Source: CAD feature listing. Evaluate the final solid. Frame: model axes, mm. A direction names the side the tool comes from. Give positions to 0.01 mm unless a question says otherwise; leave off trailing zeros. Loops run counter-clockwise (first coordinate to the right, second up) from the corner with the lowest first, then second, coordinate; pieces in that order, holes last. Notation, with made-up numbers: (19, 0.5) - (42, 0.5) arc R11 cw to (42, 9.5) - close; hole circle Ø2 at (2.25, 67.5). An arc over 180 degrees is marked (long way). Write each question's results on one line, items separated by ' | '. Start each with the question number.
(1) Reachability of faces 5 (the flat face through (20.902, 0, 2)), 6 (the flat face through (-11.536, 24, 2)), 7 (the cylindrical face through (11.998, 30.107, 1.972)), 8 (the flat face through (-27.75, 17.72, 1.97)) from +Z, -Z, +X, -X, +Y, -Y: full face, straight path, thin tool, end or side. Return the list, or none.
(2) Pull-direction query (Y, two-part tool) for faces 1 (the cylindrical face through (11.935, -30.105, 1.972)), 2 (the flat face through (-1, 1, 0)), 3 (the cylindrical face through (-36.265, -33.787, 1.972)), 4 (the cylindrical face through (-15.52, -19.77, 1.97)); classes: pulls with the +Y half, pulls with the -Y half, needs draft (parallel to the pull), parting line crosses it, or undercut.
(3) Contact query for flat-ended pins moving along their axis: pin 1 (2 mm diameter, centred on x = -3.5, z = 1.5, fed in from -Y); pin 2 (0.8 mm diameter, centred on x = -11, z = 1.5, fed in from +Y); pin 3 (0.6 mm diameter, centred on x = 10.5, z = 2, fed in from -Y). Output: stop coordinate, or through.
(4) Cut plane B-B on y = 0. Return the cut outline in (x, z).
(5) Cut plane A-A on x = 15.25. Return the cut outline in (y, z), then the cut area to 3 significant figures.
(6) Cut plane C-C on x = 5. Return the cut outline in (y, z), then the cut area to 3 significant figures.
(7) Material intervals for line 1 along X through (y, z) = (-19, 2.25); line 2 along Y through (x, z) = (-15.25, 3.1); line 3 along Y through (x, z) = (-2.5, 2.4), sorted ascending. Write a range as [from, to].
from build123d import *

# Parameters (mm, degrees)
F0_R     = 1.25
F1_DEPTH = 4


with BuildPart() as f1:
    # F0 (on Top) → F1 (new body)
    with BuildSketch(Plane.XY):
        with BuildLine():
            ThreePointArc((21.584305, 11.679198), (21.963351, 12.114397), (22.366871, 12.527004))
            Line((22.366871, 12.527004), (32.982551, 22.772845))
            ThreePointArc((32.982551, 22.772845), (33.486537, 23.413044), (33.799674, 24.165243))
            Line((33.799674, 24.165243), (34.68968, 27.534472))
            Line((34.68968, 27.534472), (36.072638, 32.76983))
            ThreePointArc((36.072638, 32.76983), (36.264823, 33.801613), (36.08985, 34.836454))
            ThreePointArc((36.08985, 34.836454), (34.783822, 36.740244), (32.927522, 38.112932))
            ThreePointArc((32.927522, 38.112932), (31.899533, 38.324475), (30.861587, 38.168982))
            Line((30.861587, 38.168982), (25.580499, 36.972463))
            Line((25.580499, 36.972463), (22.18184, 36.20244))
            ThreePointArc((22.18184, 36.20244), (21.419015, 35.916161), (20.761354, 35.435184))
            Line((20.761354, 35.435184), (20.002936, 34.703188))
            Line((20.002936, 34.703188), (18.041918, 32.81049))
            ThreePointArc((18.041918, 32.81049), (16.234056, 31.42594), (14.159835, 30.486285))
            ThreePointArc((14.159835, 30.486285), (11.966375, 30.106), (9.753047, 30.344882))
            Line((9.753047, 30.344882), (2.492354, 32.176444))
            ThreePointArc((2.492354, 32.176444), (0, 32.485953), (-2.492354, 32.176444))
            Line((-2.492354, 32.176444), (-9.753047, 30.344882))
            ThreePointArc((-9.753047, 30.344882), (-11.966375, 30.106), (-14.159835, 30.486285))
            ThreePointArc((-14.159835, 30.486285), (-16.234056, 31.42594), (-18.041918, 32.81049))
            Line((-18.041918, 32.81049), (-20.002936, 34.703188))
            Line((-20.002936, 34.703188), (-20.761354, 35.435184))
            ThreePointArc((-20.761354, 35.435184), (-21.419015, 35.916161), (-22.18184, 36.20244))
            Line((-22.18184, 36.20244), (-25.580499, 36.972463))
            Line((-25.580499, 36.972463), (-30.861587, 38.168982))
            ThreePointArc((-30.861587, 38.168982), (-31.899533, 38.324475), (-32.927522, 38.112932))
            ThreePointArc((-32.927522, 38.112932), (-34.783822, 36.740244), (-36.08985, 34.836454))
            ThreePointArc((-36.08985, 34.836454), (-36.264823, 33.801613), (-36.072638, 32.76983))
            Line((-36.072638, 32.76983), (-34.68968, 27.534472))
            Line((-34.68968, 27.534472), (-33.799674, 24.165243))
            ThreePointArc((-33.799674, 24.165243), (-33.486537, 23.413044), (-32.982551, 22.772845))
            Line((-32.982551, 22.772845), (-22.366871, 12.527004))
            ThreePointArc((-22.366871, 12.527004), (-21.963351, 12.114397), (-21.584305, 11.679198))
            ThreePointArc((-21.584305, 11.679198), (-21.078061, 10.786271), (-20.902461, 9.774951))
            Line((-20.902461, 9.774951), (-20.902461, -9.774951))
            ThreePointArc((-20.902461, -9.774951), (-21.078061, -10.786271), (-21.584305, -11.679198))
            ThreePointArc((-21.584305, -11.679198), (-21.963351, -12.114397), (-22.366871, -12.527004))
            Line((-22.366871, -12.527004), (-32.982551, -22.772845))
            ThreePointArc((-32.982551, -22.772845), (-33.486537, -23.413044), (-33.799674, -24.165243))
            Line((-33.799674, -24.165243), (-34.68968, -27.534472))
            Line((-34.68968, -27.534472), (-36.072638, -32.76983))
            ThreePointArc((-36.072638, -32.76983), (-36.264823, -33.801613), (-36.08985, -34.836454))
            ThreePointArc((-36.08985, -34.836454), (-34.783822, -36.740244), (-32.927522, -38.112932))
            ThreePointArc((-32.927522, -38.112932), (-31.899533, -38.324475), (-30.861587, -38.168982))
            Line((-30.861587, -38.168982), (-25.580499, -36.972463))
            Line((-25.580499, -36.972463), (-22.18184, -36.20244))
            ThreePointArc((-22.18184, -36.20244), (-21.419015, -35.916161), (-20.761354, -35.435184))
            Line((-20.761354, -35.435184), (-20.002936, -34.703188))
            Line((-20.002936, -34.703188), (-18.041918, -32.81049))
            ThreePointArc((-18.041918, -32.81049), (-16.234056, -31.42594), (-14.159835, -30.486285))
            ThreePointArc((-14.159835, -30.486285), (-11.966375, -30.106), (-9.753047, -30.344882))
            Line((-9.753047, -30.344882), (-2.492354, -32.176444))
            ThreePointArc((-2.492354, -32.176444), (0, -32.485953), (2.492354, -32.176444))
            Line((2.492354, -32.176444), (9.753047, -30.344882))
            ThreePointArc((9.753047, -30.344882), (11.966375, -30.106), (14.159835, -30.486285))
            ThreePointArc((14.159835, -30.486285), (16.234056, -31.42594), (18.041918, -32.81049))
            Line((18.041918, -32.81049), (20.002936, -34.703188))
            Line((20.002936, -34.703188), (20.761354, -35.435184))
            ThreePointArc((20.761354, -35.435184), (21.419015, -35.916161), (22.18184, -36.20244))
            Line((22.18184, -36.20244), (25.580499, -36.972463))
            Line((25.580499, -36.972463), (30.861587, -38.168982))
            ThreePointArc((30.861587, -38.168982), (31.899533, -38.324475), (32.927522, -38.112932))
            ThreePointArc((32.927522, -38.112932), (34.783822, -36.740244), (36.08985, -34.836454))
            ThreePointArc((36.08985, -34.836454), (36.264823, -33.801613), (36.072638, -32.76983))
            Line((36.072638, -32.76983), (34.68968, -27.534472))
            Line((34.68968, -27.534472), (33.799674, -24.165243))
            ThreePointArc((33.799674, -24.165243), (33.486537, -23.413044), (32.982551, -22.772845))
            Line((32.982551, -22.772845), (22.366871, -12.527004))
            ThreePointArc((22.366871, -12.527004), (21.963351, -12.114397), (21.584305, -11.679198))
            ThreePointArc((21.584305, -11.679198), (21.078061, -10.786271), (20.902461, -9.774951))
            Line((20.902461, -9.774951), (20.902461, 9.774951))
            ThreePointArc((20.902461, 9.774951), (21.078061, 10.786271), (21.584305, 11.679198))
        make_face()
        with Locations((-29.027586, -31.184549)):
            Circle(F0_R, mode=Mode.SUBTRACT)
        with Locations((-23.27135, -25.628853)):
            Circle(F0_R, mode=Mode.SUBTRACT)
        with BuildLine():
            ThreePointArc((-10.435595, -19.937071), (-10.152752, -20.054229), (-10.035595, -20.337071))
            Line((-10.035595, -20.337071), (-10.035595, -24.606303))
            Line((-10.035595, -24.606303), (-10.035595, -27.564576))
            ThreePointArc((-10.035595, -27.564576), (-10.152752, -27.847419), (-10.435595, -27.964576))
            Line((-10.435595, -27.964576), (-11.135595, -27.964576))
            ThreePointArc((-11.135595, -27.964576), (-11.418437, -27.847419), (-11.535595, -27.564576))
            Line((-11.535595, -27.564576), (-11.535595, -20.337071))
            ThreePointArc((-11.535595, -20.337071), (-11.418437, -20.054229), (-11.135595, -19.937071))
            Line((-11.135595, -19.937071), (-10.435595, -19.937071))
        make_face(mode=Mode.SUBTRACT)
        with Locations((-15.25, -18.549995)):
            Circle(F0_R, mode=Mode.SUBTRACT)
        with BuildLine():
            Line((11.535595, -20.337071), (11.535595, -27.564576))
            ThreePointArc((11.535595, -27.564576), (11.418437, -27.847419), (11.135595, -27.964576))
            Line((11.135595, -27.964576), (10.435595, -27.964576))
            ThreePointArc((10.435595, -27.964576), (10.152752, -27.847419), (10.035595, -27.564576))
            Line((10.035595, -27.564576), (10.035595, -24.606303))
            Line((10.035595, -24.606303), (10.035595, -20.337071))
            ThreePointArc((10.035595, -20.337071), (10.152752, -20.054229), (10.435595, -19.937071))
            Line((10.435595, -19.937071), (11.135595, -19.937071))
            ThreePointArc((11.135595, -19.937071), (11.418437, -20.054229), (11.535595, -20.337071))
        make_face(mode=Mode.SUBTRACT)
        with Locations((29.027586, -31.184549)):
            Circle(F0_R, mode=Mode.SUBTRACT)
        with Locations((23.27135, -25.628853)):
            Circle(F0_R, mode=Mode.SUBTRACT)
        with Locations((15.25, -18.549995)):
            Circle(F0_R, mode=Mode.SUBTRACT)
        with Locations((-15.25, 11.950005)):
            Circle(F0_R, mode=Mode.SUBTRACT)
        with Locations((-23.27135, 25.628853)):
            Circle(F0_R, mode=Mode.SUBTRACT)
        with Locations((-29.027586, 31.184549)):
            Circle(F0_R, mode=Mode.SUBTRACT)
        with BuildLine():
            Line((-11.135595, 27.964576), (-10.435595, 27.964576))
            ThreePointArc((-10.435595, 27.964576), (-10.152752, 27.847419), (-10.035595, 27.564576))
            Line((-10.035595, 27.564576), (-10.035595, 24.606303))
            Line((-10.035595, 24.606303), (-10.035595, 20.337071))
            ThreePointArc((-10.035595, 20.337071), (-10.152752, 20.054229), (-10.435595, 19.937071))
            Line((-10.435595, 19.937071), (-11.135595, 19.937071))
            ThreePointArc((-11.135595, 19.937071), (-11.418437, 20.054229), (-11.535595, 20.337071))
            Line((-11.535595, 20.337071), (-11.535595, 27.564576))
            ThreePointArc((-11.535595, 27.564576), (-11.418437, 27.847419), (-11.135595, 27.964576))
        make_face(mode=Mode.SUBTRACT)
        with Locations((15.25, 11.950005)):
            Circle(F0_R, mode=Mode.SUBTRACT)
        with BuildLine():
            Line((10.035595, 24.606303), (10.035595, 27.564576))
            ThreePointArc((10.035595, 27.564576), (10.152752, 27.847419), (10.435595, 27.964576))
            Line((10.435595, 27.964576), (11.135595, 27.964576))
            ThreePointArc((11.135595, 27.964576), (11.418437, 27.847419), (11.535595, 27.564576))
            Line((11.535595, 27.564576), (11.535595, 20.337071))
            ThreePointArc((11.535595, 20.337071), (11.418437, 20.054229), (11.135595, 19.937071))
            Line((11.135595, 19.937071), (10.435595, 19.937071))
            ThreePointArc((10.435595, 19.937071), (10.152752, 20.054229), (10.035595, 20.337071))
            Line((10.035595, 20.337071), (10.035595, 24.606303))
        make_face(mode=Mode.SUBTRACT)
        with Locations((23.27135, 25.628853)):
            Circle(F0_R, mode=Mode.SUBTRACT)
        with Locations((29.027586, 31.184549)):
            Circle(F0_R, mode=Mode.SUBTRACT)
    extrude(amount=F1_DEPTH)


solid = f1.part
Ans:
1) face 5: +Z, -Z, +X | face 6: +Z, -Z | face 7: +Z, -Z, +Y | face 8: +Z, -Z, -X
2) face 1: pulls with the -Y half | face 2: needs draft | face 3: undercut | face 4: undercut
3) pin 1: y = -32.17 | pin 2: y = 30.18 | pin 3: y = -30.25
4) outline: (-20.9, 0) - (20.9, 0) - (20.9, 4) - (-20.9, 4) - close
5) outline: (-30.91, 0) - (-19.8, 0) - (-19.8, 4) - (-30.91, 4) - close; (-17.3, 0) - (10.7, 0) - (10.7, 4) - (-17.3, 4) - close; (13.2, 0) - (30.91, 0) - (30.91, 4) - (13.2, 4) - close | area: 227 mm^2
6) outline: (-31.54, 0) - (31.54, 0) - (31.54, 4) - (-31.54, 4) - close | area: 252 mm^2
7) line 1: [-29.07, -16.42], [-14.08, 14.08], [16.42, 29.07] | line 2: [-30.91, -19.8], [-17.3, 10.7], [13.2, 30.91] | line 3: [-32.17, 32.17]
